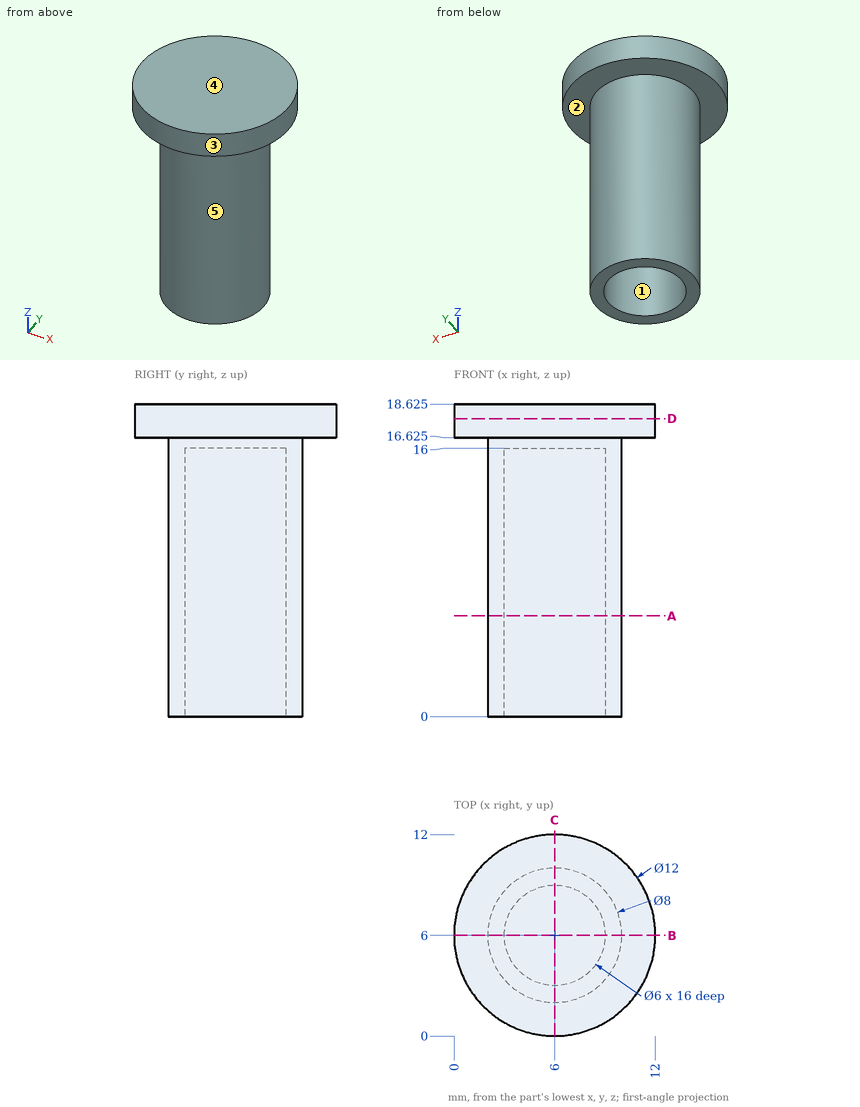
Here's the drawing with two shaded views (mm, measured from the low corner). I have some questions. A direction names the side the tool comes from. Give positions to 0.01 mm unless a question says otherwise; leave off trailing zeros. Write each loop counter-clockwise with the first axis right and the second up, starting at its lowest first coordinate (ties: lowest second). Pieces come first, ordered by that corner, then holes. Notation, with made-up numbers: (9, -18) -> (62, -18) arc R25 cw to (62, 7) -> close; hole circle Ø2 at (80, 49.5). An arc over 180 degrees is marked (long way). One line per item, written item: value.
Q1. Imagine slicing it at D-D on z = 17.75. Please give me the cut outline in (x, y).
Results found:
outline: circle Ø12 at (6, 6)
Q2. Imagine slicing it at A-A on z = 6. Please give me the cut outline in (x, y), and give its area (3 significant figures).
Results found:
outline: circle Ø8 at (6, 6); hole circle Ø6 at (6, 6)
area: 22.0 mm^2
Q3. Which directions (+Z, -Z, +X, -X, +Y, -Y) give clear straight access to the entire face, cutting with the end or side of a thin tool? Please do the marked faces 4 and 5.
Results found:
face 4: +Z, +X, -X, +Y, -Y
face 5: -Z
Q4. Please list where these lines run through material, in increasing order: line 1 (Y direction, x = 6, z = 6.25); line 2 (Z direction, x = 3, y = 9.25) (1 decimal); line 3 (X direction, y = 8, z = 13.25) (1 decimal). Write a range as [from, to].
Results found:
line 1: y = [2, 3], [9, 10]
line 2: z = [16.6, 18.6]
line 3: x = [2.5, 3.8], [8.2, 9.5]
Q5. Imagine slicing it at B-B on y = 6. Please give me the cut outline in (x, z) (1 decimal).
Results found:
outline: (0, 16.6) -> (2, 16.6) -> (2, 0) -> (3, 0) -> (3, 16) -> (9, 16) -> (9, 0) -> (10, 0) -> (10, 16.6) -> (12, 16.6) -> (12, 18.6) -> (0, 18.6) -> close
Q6. For P1, Ø1, axis at x = 5, y = 7, coming from the -Z side; P2, Ø3, axis at y = 9.5, z = 9, coming from the -X side (1 decimal); P3, Ø1, axis at x = 3, z = 8, coming from the -Y side, each with a flat end and sliding along its axis, tell me the tip position at first contact or that it passes through.
Results found:
P1: stops at z = 16
P2: stops at x = 2.5
P3: stops at y = 2.88
Q7. We'd pull the mould along X, two halves only. Please class the marked faces 1, 2 and 3: +X half, -X half, draft (parallel to the pull), parting line (faces both ways), or undercut.
Results found:
face 1: undercut
face 2: draft
face 3: parting line
